from build123d import *

# Parameters (mm, degrees)
SKETCH1_W           = 100
SKETCH1_H           = 80
BOSS_EXTRUDE1_DEPTH = 3
BOSS_EXTRUDE2_DEPTH = 31.1
BOSS_EXTRUDE3_DEPTH = 65
SKETCH4_R           = 3
SKETCH4_R_2         = 1.425
BOSS_EXTRUDE4_DEPTH = 5
LPATTERN1_COUNT     = 2
LPATTERN1_PITCH     = 44.6
CUT_EXTRUDE1_DEPTH  = 111.325926237


with BuildPart() as part:
    # Sketch1 → Boss-Extrude1 (new body)
    with BuildSketch(Plane(origin=(0, 0, 0), x_dir=(1, 0, 0), z_dir=(0, 1, 0))):
        Rectangle(SKETCH1_W, SKETCH1_H)
    extrude(amount=BOSS_EXTRUDE1_DEPTH)

    # Sketch2 → Boss-Extrude2 (add)
    with BuildSketch(Plane(origin=(0, 3, 0), x_dir=(1, 0, 0), z_dir=(0, 1, 0))):
        Polygon((-50, 40), (50, 40), (50, -40), (47, -40), (47, 37), (-47, 37), (-47, -40), (-50, -40), align=None)
    extrude(amount=BOSS_EXTRUDE2_DEPTH)

    # Sketch3 → Boss-Extrude3 (add)
    with BuildSketch(Plane.XY.offset(-37)):
        with BuildLine():
            Line((47, 26), (37, 26))
            ThreePointArc((37, 26), (27.807611845, 22.192388155), (24, 13))
            Line((24, 13), (24, 3))
            Line((24, 3), (37, 3))
            ThreePointArc((37, 3), (29.928932188, 20.071067812), (47, 13))
            Line((47, 13), (47, 26))
        make_face()
        with BuildLine():
            Line((47, 3), (47, 13))
            ThreePointArc((47, 13), (44.071067812, 5.928932188), (37, 3))
            Line((37, 3), (47, 3))
        make_face()
    extrude(amount=BOSS_EXTRUDE3_DEPTH)

    # Sketch4 → Boss-Extrude4 (add)
    with BuildSketch(Plane(origin=(0, 3, 0), x_dir=(1, 0, 0), z_dir=(0, 1, 0))):
        with Locations(Location((18, 22, 0), (0, 0, 90))):
            Circle(SKETCH4_R)
        with Locations(Location((18, 22, 0), (0, 0, 270))):
            Circle(SKETCH4_R_2, mode=Mode.SUBTRACT)
    boss_extrude4 = extrude(amount=BOSS_EXTRUDE4_DEPTH)

    # LPattern1: Boss-Extrude4 ×2
    with Locations(*[(0, 0, i * LPATTERN1_PITCH) for i in range(1, LPATTERN1_COUNT)]):
        add(boss_extrude4)

    # Sketch10 → Cut-Extrude1 (cut, through all)
    with BuildSketch(Plane.ZY.offset(-47)):
        with BuildLine():
            Line((-10, 29), (10, 29))
            ThreePointArc((10, 29), (11, 28), (10, 27))
            Line((10, 27), (-10, 27))
            ThreePointArc((-10, 27), (-11, 28), (-10, 29))
        make_face()
    extrude(amount=-CUT_EXTRUDE1_DEPTH, mode=Mode.SUBTRACT)


solid = part.part
Design review of the part built by this model. Coordinates are the model's own, in mm. A direction names the side the tool comes from. Give positions to 0.01 mm unless a question says otherwise; leave off trailing zeros. Write each loop counter-clockwise with the first axis right and the second up, starting at its lowest first coordinate (ties: lowest second). Pieces come first, ordered by that corner, then holes. Notation, with made-up numbers: M 24,31 L 44,31 A9 ccw 44,48 Z; hole C -14.75,37.25 d6. An arc over 180 degrees is marked long. Return JSON: item names as keys, results as strings. Group by question number.
Item 1: Tool access review of faces 4 (the flat face through (37, 13, -37)), 5 (the flat face through (48, 27, 0)), 6 (the cylindrical face through (16.61, 5.46, 22.29)), 7 (the flat face through (-47, 18, 1)): name each direction out of +Z, -Z, +X, -X, +Y, -Y from which nothing blocks a thin tool from reaching the whole face with its end or side.
Item 2: Wall thickness on line 1 along X through (y, z) = (30, 23.5); line 2 along Y through (x, z) = (37, 2); line 3 along X through (y, z) = (9, -13): over which ranges is each line inside the solid? List them lowest first.
Item 3: Take a section at C-C (y = 21.5). Give the boundary of the cut face in (x, z).
Item 4: Take a section at D-D (x = -6). Give the boundary of the cut face in (y, z), plus the area to 3 significant figures.
Item 5: Take a section at A-A (z = -7.5). Give the boundary of the cut face in (x, y), plus the area to 3 significant figures.
Item 6: Take a section at B-B (z = 22.6). Give the boundary of the cut face in (x, y) (3 decimals).
Item 7: The part is to be moulded in two halves that separate along X. For faces 1 (the flat face through (24, 8, -5)), 2 (the flat face through (0, 34.1, -39)), 3 (the flat face through (50, 17, -1)), say which applies: pulls with the +X half, pulls with the -X half, needs draft (parallel to the pull), parting line crosses it, or undercut.
Item 8: Clearance check with flat-ended pins moving along their axes: pin 1 Ø4 at (x, z) = (-14.5, -3.5) entering from +Y; pin 2 Ø5 at (x, y) = (40.5, 10) entering from +Z; pin 3 Ø3 at (x, z) = (40.5, -15.5) entering from +Y. State where each tip first meets the part, or that it passes through.
Return value:
{
 "1": {"face 4": "+Z", "face 5": "+X", "face 6": "+Y", "face 7": "+Z, +Y"},
 "2": {"line 1": "x = -50 to -47, 47 to 50", "line 2": "y = 0 to 3, 23 to 26", "line 3": "x = -50 to -47, 24 to 27.83, 46.17 to 50"},
 "3": {"outline": "M -50,-40 L 50,-40 L 50,40 L 47,40 L 47,28 L 42.27,28 L 42.27,-37 L 31.73,-37 L 31.73,28 L 27.16,28 L 27.16,-37 L -47,-37 L -47,40 L -50,40 Z"},
 "4": {"outline": "M 0,-40 L 34.1,-40 L 34.1,-37 L 3,-37 L 3,40 L 0,40 Z", "area": "333 mm2"},
 "5": {"outline": "M -50,0 L 50,0 L 50,27 L 47,27 L 47,26 L 37,26 A13 ccw 24,13 L 24,3 L -47,3 L -47,34.1 L -50,34.1 Z; M 47,29 L 50,29 L 50,34.1 L 47,34.1 Z; hole C 37,13 d20", "area": "659 mm2"},
 "6": {"outline": "M -50,0 L 50,0 L 50,34.1 L 47,34.1 L 47,26 L 37,26 A13 ccw 24,13 L 24,3 L 21,3 L 21,8 L 19.425,8 L 19.425,3 L 16.575,3 L 16.575,8 L 15,8 L 15,3 L -47,3 L -47,34.1 L -50,34.1 Z; hole C 37,13 d20"},
 "7": {"face 1": "undercut", "face 2": "needs draft", "face 3": "pulls with the +X half"},
 "8": {"pin 1": "stops at y = 3", "pin 2": "stops at z = -37", "pin 3": "stops at y = 26"}
}
